Geometry: final body of the model. Coordinates: model frame, mm. A direction names the side the tool comes from. Round coordinates to 2 decimals unless told otherwise and drop trailing zeros. Loops run counter-clockwise (first coordinate to the right, second up) from the corner with the lowest first, then second, coordinate; pieces in that order, holes last. Notation, with made-up numbers: (22, 18) - (47, 18) arc R17 cw to (47, 28) - close; hole circle Ø4 at (84.5, 11.25). An arc over 180 degrees is marked (long way). Write item = value, one per line. Start each with the question number.
Item 1: Line query: line 1 (Y direction, x = 0, z = 17.25); line 2 (Z direction, x = -5, y = 0.75); line 3 (X direction, y = -1.5, z = 21). Output: solid intervals per line, ascending. Write a range as from..to.
Item 2: First-contact query: pin 1 (5 mm diameter, centred on y = -4, z = 13, fed in from +X); pin 2 (2 mm diameter, centred on x = 2, z = 13.5, fed in from -Y); pin 3 (1.5 mm diameter, centred on y = -1, z = 5.5, fed in from +X). Flat tips, straight axial feed; report the tip coordinate or a pass-through.
Item 3: Section A-A (x = 0). Return loops of the section in (y, z).
Item 4: Section C-C (x = -2). Return loops of the section in (y, z).
Item 5: Access query for faces 1 (the cylindrical face through (1.03, 4.65, 33.21)), 2 (the flat face through (-2, 2, 38.1)). Directions: +Z, -Z, +X, -X, +Y, -Y. A direction counts if a zero-diameter tool reaches every point of the face in a straight line with its end or side. Return the directions, or none.
Item 6: Section D-D (z = 25.5). Return loops of the section in (x, y) (1 decimal).
Item 7: Section B-B (z = 36). Return loops of the section in (x, y) (1 decimal).
from build123d import *

# Parameters (mm, degrees)
SKETCH2_R                   = 7.9375
CYLINDER_BASE_DEPTH         = 38.1
TRIM_1_DEPTH                = 40.71923731
TRIM_1_DEPTH_BACK           = 9.652
SKETCH3_OUTSIDE_W           = 26.72
SKETCH3_OUTSIDE_H           = 26.72
SKETCH3_OUTSIDE_R           = 4.7625
F_1_4_20_TAPPED_HOLE1_D     = 5.1054
F_1_4_20_TAPPED_HOLE1_DEPTH = 17.516183098
F_1_4_20_TAPPED_HOLE1_TIP   = 1.533816902
F_1_4_20_TAPPED_HOLE9_D     = 5.1054
F_1_4_20_TAPPED_HOLE9_DEPTH = 12.436183098
F_1_4_20_TAPPED_HOLE9_TIP   = 1.533816902
SKETCH20_R                  = 2.5527
CUT_EXTRUDE2_DEPTH          = 40.71923731


with BuildPart() as part:
    # Sketch2 → Cylinder Base (new body)
    with BuildSketch(Plane.XY):
        with Locations(Location((0, 0, 0), (0, 0, 180))):
            Circle(SKETCH2_R)
    extrude(amount=CYLINDER_BASE_DEPTH)

    # Sketch3 outside → Trim 1 (cut, two sides: drawn at the far end of the back side and taken through both)
    with BuildSketch(Plane.XY.offset(38.1).offset(-TRIM_1_DEPTH_BACK)):
        Rectangle(SKETCH3_OUTSIDE_W, SKETCH3_OUTSIDE_H)
        with Locations(Location((0, 0, 0), (0, 0, 180))):
            Circle(SKETCH3_OUTSIDE_R, mode=Mode.SUBTRACT)
    extrude(amount=TRIM_1_DEPTH + TRIM_1_DEPTH_BACK, mode=Mode.SUBTRACT)

    # 1/4-20 Tapped Hole1
    with Locations(Plane.XY.offset(38.1)):
        with Locations((0, 0)):
            Hole(F_1_4_20_TAPPED_HOLE1_D / 2, depth=F_1_4_20_TAPPED_HOLE1_DEPTH)
            with Locations((0, 0, -(F_1_4_20_TAPPED_HOLE1_DEPTH + F_1_4_20_TAPPED_HOLE1_TIP / 2))):  # 118° drill point
                Cone(0, F_1_4_20_TAPPED_HOLE1_D / 2, F_1_4_20_TAPPED_HOLE1_TIP, mode=Mode.SUBTRACT)

    # 1/4-20 Tapped Hole9
    with Locations(Plane(origin=(0, 0, 0), x_dir=(-1, 0, 0), z_dir=(0, 0, -1))):
        with Locations((0, 0)):
            Hole(F_1_4_20_TAPPED_HOLE9_D / 2, depth=F_1_4_20_TAPPED_HOLE9_DEPTH)
            with Locations((0, 0, -(F_1_4_20_TAPPED_HOLE9_DEPTH + F_1_4_20_TAPPED_HOLE9_TIP / 2))):  # 118° drill point
                Cone(0, F_1_4_20_TAPPED_HOLE9_D / 2, F_1_4_20_TAPPED_HOLE9_TIP, mode=Mode.SUBTRACT)

    # Sketch20 → Cut-Extrude2 (cut, through all)
    with BuildSketch(Plane.XY.offset(38.1)):
        Circle(SKETCH20_R)
    extrude(amount=-CUT_EXTRUDE2_DEPTH, mode=Mode.SUBTRACT)


solid = part.part
Taken from the geometry:
q1.line_1 = -7.94..-2.55, 2.55..7.94
q1.line_2 = 0..28.45
q1.line_3 = -7.79..-2.07, 2.07..7.79
q2.pin_1 = 7.79
q2.pin_2 = -7.87
q2.pin_3 = 7.93
q3.outline = (-7.94, 0) - (-2.55, 0) - (-2.55, 38.1) - (-4.76, 38.1) - (-4.76, 28.45) - (-7.94, 28.45) - close; (2.55, 0) - (7.94, 0) - (7.94, 28.45) - (4.76, 28.45) - (4.76, 38.1) - (2.55, 38.1) - close
q4.outline = (-7.68, 0) - (-1.59, 0) - (-1.59, 38.1) - (-4.32, 38.1) - (-4.32, 28.45) - (-7.68, 28.45) - close; (1.59, 0) - (7.68, 0) - (7.68, 28.45) - (4.32, 28.45) - (4.32, 38.1) - (1.59, 38.1) - close
q5.face_1 = +Z
q5.face_2 = +Z, +X, -X, +Y, -Y
q6.outline = circle Ø15.9 at (0, 0); hole circle Ø5.1 at (0, 0)
q7.outline = circle Ø9.5 at (0, 0); hole circle Ø5.1 at (0, 0)
